from build123d import *

# Parameters (mm, degrees)
F2_DEPTH = 273.05
F3_SIZE  = 1.5


with BuildPart() as f2:
    # F1 (on Top) → F2 (new body)
    with BuildSketch(Plane.XY):
        with BuildLine():
            Line((18.3301270189, -5.5829037687), (4.3301270189, 18.6658075373))
            ThreePointArc((4.3301270189, 18.6658075373), (0, 21.1658075373), (-4.3301270189, 18.6658075373))
            Line((-4.3301270189, 18.6658075373), (-18.3301270189, -5.5829037687))
            ThreePointArc((-18.3301270189, -5.5829037687), (-18.3301270189, -10.5829037687), (-14, -13.0829037687))
            Line((-14, -13.0829037687), (14, -13.0829037687))
            ThreePointArc((14, -13.0829037687), (18.3301270189, -10.5829037687), (18.3301270189, -5.5829037687))
        make_face()
    extrude(amount=F2_DEPTH)

    # F3
    f3_edges = [f2.edges().sort_by_distance(p)[0] for p in [
        (11.330127, 6.541452, 273.05),
        (0, 21.165808, 273.05),
        (-11.330127, 6.541452, 273.05),
        (-18.330127, -10.582904, 273.05),
        (0, -13.082904, 273.05),
        (18.330127, -10.582904, 273.05),
    ]]
    chamfer(f3_edges, length=F3_SIZE)


solid = f2.part
Can you work these out from the model? Positions are in its coordinate system, mm. Coordinates: 2 decimals unless noted, no trailing zeros. Loops run counter-clockwise (first coordinate to the right, second up) from the corner with the lowest first, then second, coordinate; pieces in that order, holes last. Notation, with made-up numbers: (39.25, -36) - (97.25, -36) arc R18 cw to (97.25, -26) - close; hole circle Ø2 at (80.25, 38). An arc over 180 degrees is marked (long way). Answer as a JSON object with one key per item and string values. Group by question number.
Item 1: If we section it at B-B (y = 5.5): List the corners of the cut face in (x, z) for me, plus the area to 3 significant figures.
Item 2: If we section it at A-A (z = 77): List the corners of the cut face in (x, y) for me.
Item 3: If I drill on L1, parallel to Y at x = 7, z = 30.5; L2, parallel to Y at x = -8.5, z = 64.5; L3, parallel to X at y = 18, z = 116, over which ranges is the centre line in solid material (lowest first)? Write a range as from..to.
Item 4: For pin 1 (1 mm diameter, centred on x = 9, y = 13, fed in from +Z); pin 2 (3 mm diameter, centred on y = -4, z = 77.5, fed in from -X); pin 3 (1 mm diameter, centred on y = -1, z = 54.5, fed in from +X); pin 4 (1.5 mm diameter, centred on y = 12.5, z = 209.5, fed in from -X), each with a flat end and sliding along its axis, tell me the tip position at first contact or that it passes through.
Returned:
{
 "1": {"outline": "(-11.93, 0) - (11.93, 0) - (11.93, 271.55) - (10.2, 273.05) - (-10.2, 273.05) - (-11.93, 271.55) - close", "area": "6,510 mm²"},
 "2": {"outline": "(-18.33, -5.58) arc R5 ccw to (-14, -13.08) - (14, -13.08) arc R5 ccw to (18.33, -5.58) - (4.33, 18.67) arc R5 ccw to (-4.33, 18.67) - close"},
 "3": {"L1": "y = -13.08..14.04", "L2": "y = -13.08..11.44", "L3": "x = -4.71..4.71"},
 "4": {"pin 1": "passes through", "pin 2": "stops at x = -18.28", "pin 3": "stops at x = 15.97", "pin 4": "stops at x = -8.32"}
}
